Could you check a few things on this model? Use its own coordinates, in mm. A direction names the side the tool comes from. Coordinates: 2 decimals unless noted, no trailing zeros. Write each loop counter-clockwise with the first axis right and the second up, starting at its lowest first coordinate (ties: lowest second). Pieces come first, ordered by that corner, then holes. Notation, with made-up numbers: (10, 47) - (26, 47) arc R26 cw to (26, 65) - close; hole circle Ø1 at (-24.5, 8.5). An arc over 180 degrees is marked (long way). Answer as a JSON object with one key per item and string values. Group by question number.
1) If we section it at D-D (z = 5.5): Write out the boundary of the cut face in (x, y).
2) If we section it at C-C (y = 21): Write out the boundary of the cut face in (x, z).
3) Please list where these lines run through material, in increasing order: line 1 along Y through (x, z) = (37.5, 7); line 2 along Y through (x, z) = (4.5, 3.75); line 3 along X through (y, z) = (17.5, 0.75).
4) If we section it at A-A (x = 37.5): Write out the boundary of the cut face in (y, z), plus the area to 3 significant figures.
5) If we section it at B-B (y = 9): Write out the boundary of the cut face in (x, z), plus the area to 4 significant figures.
6) On a 3-axis mill with a long thin cutter (end or side, diameter ignored), from which of +Z, -Z, +X, -X, +Y, -Y can I reach the whole of each face in a straight line? I mean faces 5 (the flat face through (16, 15, 9)), 6 (the flat face through (36, 16, 4)). Say none if no direction works.
7) We'd pull the mould along X, two halves only. Please class faces 1 (the flat face through (30, 23, 4)), 2 (the flat face through (0, 15, 4)), 3 (the cylindrical face through (3.02, 11.32, 4.44)), 4 (the cylindrical face through (40.247, 9.121, 4.437)): released by +X, released by -X, zero draft, split by the parting line, or undercut.
8) Will this pin go through, and if not, where does the flat tip stop? pin 1 Ø5 at (x, y) = (37.5, 9) entering from +Z.
```python
from build123d import *

# Parameters (mm, degrees)
SKETCH_1_W          = 42
SKETCH_1_H          = 30
EXTRUDE_1_DEPTH     = 9
SKETCH_2_W          = 12
SKETCH_2_H          = 14
CUT_EXTRUDE_1_DEPTH = 53.39274759
CHAMFER_1_SIZE      = 0.5
SKETCH_3_R          = 2.75
CUT_EXTRUDE_2_DEPTH = 53.39274759


with BuildPart() as part:
    # 草图1 → 凸台-拉伸1 (new body)
    with BuildSketch(Plane.XY):
        with Locations((21, 15)):
            Rectangle(SKETCH_1_W, SKETCH_1_H)
    extrude(amount=EXTRUDE_1_DEPTH)

    # 草图2 → 切除-拉伸1 (cut, through all)
    with BuildSketch(Plane(origin=(0, 0, 0), x_dir=(-1, 0, 0), z_dir=(0, 0, -1))):
        with Locations((-36, 23)):
            Rectangle(SKETCH_2_W, SKETCH_2_H)
    extrude(amount=-CUT_EXTRUDE_1_DEPTH, mode=Mode.SUBTRACT)

    # 倒角1
    chamfer_1_edges = [part.edges().sort_by_distance(p)[0] for p in [
        (42, 8, 9),
        (15, 30, 0),
        (15, 30, 9),
        (42, 16, 4.5),
        (30, 23, 9),
        (30, 30, 4.5),
        (36, 16, 9),
        (36, 16, 0),
        (30, 23, 0),
        (0, 15, 9),
        (42, 8, 0),
        (21, 0, 0),
        (0, 15, 0),
        (21, 0, 9),
        (0, 30, 4.5),
        (42, 0, 4.5),
        (0, 0, 4.5),
    ]]
    chamfer(chamfer_1_edges, length=CHAMFER_1_SIZE)

    # 草图3 → 切除-拉伸2 (cut, through all)
    with BuildSketch(Plane(origin=(0, 0, 0), x_dir=(-1, 0, 0), z_dir=(0, 0, -1))):
        with Locations((-37.5, 9)):
            Circle(SKETCH_3_R)
        with Locations((-4.5, 9)):
            Circle(SKETCH_3_R)
    extrude(amount=-CUT_EXTRUDE_2_DEPTH, mode=Mode.SUBTRACT)


solid = part.part
```
Here are the results:
{
 "1": {"outline": "(0, 0.5) - (0.5, 0) - (41.5, 0) - (42, 0.5) - (42, 15.5) - (41.5, 16) - (30, 16) - (30, 29.5) - (29.5, 30) - (0.5, 30) - (0, 29.5) - close; hole circle Ø5.5 at (4.5, 9); hole circle Ø5.5 at (37.5, 9)"},
 "2": {"outline": "(0, 0.5) - (0.5, 0) - (29.5, 0) - (30, 0.5) - (30, 8.5) - (29.5, 9) - (0.5, 9) - (0, 8.5) - close"},
 "3": {"line 1": "y = 0 to 6.25, 11.75 to 16", "line 2": "y = 0 to 6.25, 11.75 to 30", "line 3": "x = 0 to 30"},
 "4": {"outline": "(0, 0.5) - (0.5, 0) - (6.25, 0) - (6.25, 9) - (0.5, 9) - (0, 8.5) - close; (11.75, 0) - (15.5, 0) - (16, 0.5) - (16, 8.5) - (15.5, 9) - (11.75, 9) - close", "area": "94.0 mm²"},
 "5": {"outline": "(0, 0.5) - (0.5, 0) - (1.75, 0) - (1.75, 9) - (0.5, 9) - (0, 8.5) - close; (7.25, 0) - (34.75, 0) - (34.75, 9) - (7.25, 9) - close; (40.25, 0) - (41.5, 0) - (42, 0.5) - (42, 8.5) - (41.5, 9) - (40.25, 9) - close", "area": "278.5 mm²"},
 "6": {"face 5": "+Z, +X, -X, +Y, -Y", "face 6": "+Z, -Z, +X, +Y"},
 "7": {"face 1": "released by +X", "face 2": "released by -X", "face 3": "undercut", "face 4": "undercut"},
 "8": {"pin 1": "passes through"}
}
